Work out the finished part from the listing and answer in its coordinate system (mm). Face numbers are marked on the shaded views. Give positions to 0.01 mm unless a question says otherwise; leave off trailing zeros. Loops run counter-clockwise (first coordinate to the right, second up) from the corner with the lowest first, then second, coordinate; pieces in that order, holes last. Notation, with made-up numbers: (20.25, 52.25) -> (24.25, 52.25) arc R32 cw to (24.25, 84.25) -> close; hole circle Ø1 at (49.5, 62.25). An arc over 180 degrees is marked (long way). Answer as CSV lines item,"result". Start each with the question number.
1. Find the intervals of material crossed by line 1 along X through (y, z) = (13.25, 8); line 2 along X through (y, z) = (5.75, 5); line 3 along Z through (x, y) = (0.25, 23.75), in increasing order.
2. Find section C-C, the plane z = 9. Give the vertices of the cut face in (x, y), and give its area (3 significant figures).
3. Determine the mould class of the marked faces 1, 2 and 3 for opening direction X: +X half, -X half, draft (parallel to the pull), parting line (faces both ways), or undercut.
4. Find section D-D, the plane x = 0. Give the vertices of the cut face in (y, z).
5. Find section A-A, the plane z = 2.25. Give the vertices of the cut face in (x, y).
6. Flat-ended cylindrical pins translate along their axes: pin 1 Ø2 at (x, y) = (-8, 21.5) entering from -Z; pin 2 Ø8 at (x, y) = (7, 14) entering from -Z; pin 3 Ø2 at (y, z) = (4.5, 3) entering from -X. Find the tip coordinate at first contact, or state that the pin passes through.
from build123d import *

# Parameters (mm, degrees)
EXTRUDE_1_DEPTH = 25
FILLET_2_R      = 1


with BuildPart() as part:
    # Эскиз1 → Бобышка-Вытянуть1 (new body)
    with BuildSketch(Plane(origin=(0, 0, 0), x_dir=(1, 0, 0), z_dir=(0, 1, 0))):
        with BuildLine():
            Line((-12.459935794, 0), (-11.456439237, 0))
            ThreePointArc((-11.456439237, 0), (-10.780775313, -0.262790219), (-10.46022713, -0.913043478))
            ThreePointArc((-10.46022713, -0.913043478), (0.456954668, -10.49005207), (10.5, 0))
            Line((10.5, 0), (13.5, 0))
            ThreePointArc((13.5, 0), (0.540433214, -13.489178327), (-13.456730658, -1.08))
            ThreePointArc((-13.456730658, -1.08), (-13.194782717, -0.321767002), (-12.459935794, 0))
        make_face()
    extrude(amount=EXTRUDE_1_DEPTH)

    # Скругление2
    fillet_2_edges = [part.edges().sort_by_distance(p)[0] for p in [
        (10.5, 12.5, 0),
        (13.5, 12.5, 0),
    ]]
    fillet(fillet_2_edges, radius=FILLET_2_R)


solid = part.part
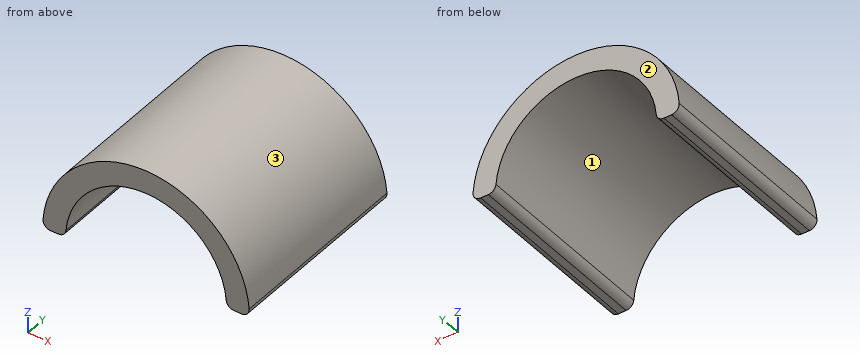
Resolved:
1,line 1,"x = -10.87 to -6.8, 6.8 to 10.87"
1,line 2,"x = -12.54 to -9.23, 9.23 to 12.54"
1,line 3,"z = 10.5 to 13.5"
2,outline,"(-10.06, 0) -> (-5.41, 0) -> (-5.41, 25) -> (-10.06, 25) -> close; (5.41, 0) -> (10.06, 0) -> (10.06, 25) -> (5.41, 25) -> close"
2,area,"233 mm^2"
3,face 1,"undercut"
3,face 2,"draft"
3,face 3,"parting line"
4,outline,"(0, 10.5) -> (25, 10.5) -> (25, 13.5) -> (0, 13.5) -> close"
5,outline,"(-13.31, 0) -> (-10.26, 0) -> (-10.26, 25) -> (-13.31, 25) -> close; (10.26, 0) -> (13.31, 0) -> (13.31, 25) -> (10.26, 25) -> close"
6,pin 1,"stops at z = 5.41"
6,pin 2,"stops at z = 0.11"
6,pin 3,"stops at x = -13.35"
